Work out the finished part from the listing and answer in its coordinate system (mm). Coordinates: 2 decimals unless noted, no trailing zeros. Order: outer loops, then holes, each group sorted by start corner. A loop starts at its lowest first (then second) coordinate and runs counter-clockwise, first axis right, second up. Notation, with made-up numbers: M 52.5,62.5 L 60.5,62.5 A20 cw 60.5,95.5 Z; hole C 55.25,74.5 d10. An arc over 180 degrees is marked long. Write item = value, one per line. Start each with the question number.
Q1. Each of these flat-tipped pins is pushed along its axis until it touches: P1, Ø1, axis at y = -1.5, z = 1, coming from the -X side; P2, Ø1, axis at y = 1, z = 1.5, coming from the -X side. Where does it stop, or does it pass through?
Q2. Find section B-B on z = 0.7. Give the vertices of the cut face in (x, y).
Q3. Find section A-A on x = -18. Give the vertices of the cut face in (y, z), and give its area (3 significant figures).
Q4. Find section D-D on y = 2. Give the vertices of the cut face in (x, z), and give its area (3 significant figures).
Q5. Find section C-C on x = 10.5. Give the vertices of the cut face in (y, z), and give its area (3 significant figures).
Q6. Straight lines are drawn through the part: line 1 along X through (y, z) = (-6.5, 1.25); line 2 along X through (y, z) = (-6.25, 0.7); line 3 along Y through (x, z) = (20.5, 2.6). For each, find the intervals that lie inside material, in ascending order.
```python
from build123d import *

# Parameters (mm, degrees)
ESBO_O1_R                = 2.458273609
ESBO_O1_R_2              = 2.41299998
RESSALTO_EXTRUS_O2_DEPTH = 3


with BuildPart() as part:
    # Esboço1 → Ressalto-extrusão2 (new body)
    with BuildSketch(Plane.XY):
        Polygon((-3.440879294, 5.164211145), (0.023622001, 5.620321217), (0.023622001, -21.15127821), (-3.440879351, -20.69516813), (-20.982927009, -12.254172046), (-22.056381633, -11.43048149), (-22.880072189, -10.357026984), (-23.397865785, -9.106962052), (-23.598378589, -7.765478496), (-23.397865785, -6.423994009), (-22.880072189, -5.173929077), (-22.056381633, -4.100475502), (-20.982927009, -3.276784015), align=None)
        with Locations((-18.391378755, -7.765478496)):
            Circle(ESBO_O1_R, mode=Mode.SUBTRACT)
        Polygon((0.023622001, 5.620321217), (3.488123295, 5.164211145), (21.030171011, -3.276784015), (22.103625634, -4.100475502), (22.92731619, -5.173929077), (23.445109786, -6.423994009), (23.645622591, -7.765478496), (23.445109786, -9.106962052), (22.92731619, -10.357026984), (22.103625634, -11.43048149), (21.030171011, -12.254172046), (3.488123352, -20.69516813), (0.023622001, -21.15127821), align=None)
        with Locations((18.438620428, -7.765478496)):
            Circle(ESBO_O1_R_2, mode=Mode.SUBTRACT)
    extrude(amount=RESSALTO_EXTRUS_O2_DEPTH)


solid = part.part
```
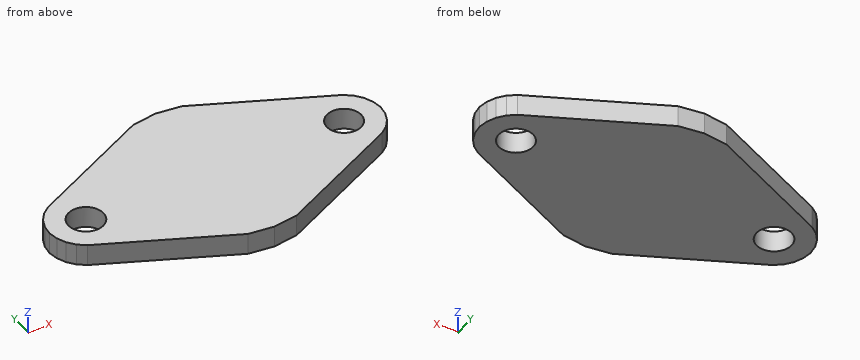
Findings below:
q1.P1 = -18.33
q1.P2 = -13.13
q2.outline = M -23.6,-7.77 L -23.4,-9.11 L -22.88,-10.36 L -22.06,-11.43 L -20.98,-12.25 L -3.44,-20.7 L 0.02,-21.15 L 3.49,-20.7 L 21.03,-12.25 L 22.1,-11.43 L 22.93,-10.36 L 23.45,-9.11 L 23.65,-7.77 L 23.45,-6.42 L 22.93,-5.17 L 22.1,-4.1 L 21.03,-3.28 L 3.49,5.16 L 0.02,5.62 L -3.44,5.16 L -20.98,-3.28 L -22.06,-4.1 L -22.88,-5.17 L -23.4,-6.42 Z; hole C -18.39,-7.77 d4.92; hole C 18.44,-7.77 d4.83
q3.outline = M -13.69,0 L -10.19,0 L -10.19,3 L -13.69,3 Z; M -5.34,0 L -1.84,0 L -1.84,3 L -5.34,3 Z
q3.area = 21.0 mm^2
q4.outline = M -10.02,0 L 10.06,0 L 10.06,3 L -10.02,3 Z
q4.area = 60.2 mm^2
q5.outline = M -17.32,0 L 1.79,0 L 1.79,3 L -17.32,3 Z
q5.area = 57.3 mm^2
q6.line_1 = -23.41 to -20.5, -16.28 to 16.38, 20.49 to 23.46
q6.line_2 = -23.33 to -20.33, -16.46 to 16.56, 20.32 to 23.37
q6.line_3 = -12.51 to -9.02, -6.51 to -3.02
